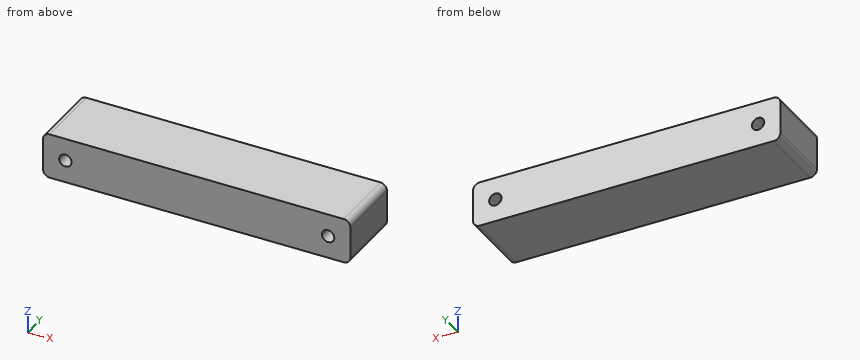
from build123d import *

# Parameters (mm, degrees)
BOSS_EXTRUDE1_DEPTH      = 30.2
M5_CLEARANCE_HOLE1_D     = 5.5
M5_CLEARANCE_HOLE1_DEPTH = 30.2


with BuildPart() as part:
    # Sketch1 → Boss-Extrude1 (new body)
    with BuildSketch(Plane(origin=(0, 0, 0), x_dir=(1, 0, 0), z_dir=(0, 1, 0))):
        with BuildLine():
            Line((65, -10), (-65, -10))
            ThreePointArc((-65, -10), (-67.121320344, -9.121320344), (-68, -7))
            Line((-68, -7), (-68, 7))
            ThreePointArc((-68, 7), (-67.121320344, 9.121320344), (-65, 10))
            Line((-65, 10), (65, 10))
            ThreePointArc((65, 10), (67.121320344, 9.121320344), (68, 7))
            Line((68, 7), (68, -7))
            ThreePointArc((68, -7), (67.121320344, -9.121320344), (65, -10))
        make_face()
    extrude(amount=BOSS_EXTRUDE1_DEPTH)

    # M5 Clearance Hole1
    with Locations(Plane(origin=(0, 30.2, 0), x_dir=(1, 0, 0), z_dir=(0, 1, 0))):
        with Locations((-58.1, 0), (58.1, 0)):
            Hole(M5_CLEARANCE_HOLE1_D / 2, depth=M5_CLEARANCE_HOLE1_DEPTH)


solid = part.part
Check sheet for the modelled part. Datum: model origin and axes. Units: mm. Give positions to 0.01 mm unless a question says otherwise; leave off trailing zeros. Write each loop counter-clockwise with the first axis right and the second up, starting at its lowest first coordinate (ties: lowest second). Pieces come first, ordered by that corner, then holes. Notation, with made-up numbers: (47.5, -24) -> (51.5, -24) arc R34 ccw to (51.5, 13) -> close; hole circle Ø6 at (36, 78.5). An arc over 180 degrees is marked (long way). Write item = value, one per line.
Item 1: Sectioned sample at B-B on x = -58.1. Record the boundary of the cut face in (y, z), and give its area (3 significant figures).
Output:
outline = (0, -10) -> (30.2, -10) -> (30.2, -2.75) -> (0, -2.75) -> close; (0, 2.75) -> (30.2, 2.75) -> (30.2, 10) -> (0, 10) -> close
area = 438 mm^2
Item 2: Scan lines: probe 1 along Z at (x, y) = (58, 20); probe 2 along X at (y, z) = (23, -2.25); probe 3 along X at (y, z) = (27.5, 7.25). Record each from-to range of solid material in increasing order. Write a range as from..to.
Output:
probe_1 = -10..-2.75, 2.75..10
probe_2 = -68..-59.68, -56.52..56.52, 59.68..68
probe_3 = -67.99..67.99
Item 3: Sectioned sample at C-C on y = 18.5. Record the boundary of the cut face in (x, z).
Output:
outline = (-68, -7) arc R3 ccw to (-65, -10) -> (65, -10) arc R3 ccw to (68, -7) -> (68, 7) arc R3 ccw to (65, 10) -> (-65, 10) arc R3 ccw to (-68, 7) -> close; hole circle Ø5.5 at (-58.1, 0); hole circle Ø5.5 at (58.1, 0)
Item 4: Gauge pin test, flat end, axial feed: pin 1 (6.5 mm diameter, centred on x = -58.1, z = 0, fed in from +Y). Record the tip position at first contact, or that the pin passes through.
Output:
pin_1 = 30.2
Item 5: Sectioned sample at A-A on z = 0. Record the boundary of the cut face in (x, y).
Output:
outline = (-68, 0) -> (-60.85, 0) -> (-60.85, 30.2) -> (-68, 30.2) -> close; (-55.35, 0) -> (55.35, 0) -> (55.35, 30.2) -> (-55.35, 30.2) -> close; (60.85, 0) -> (68, 0) -> (68, 30.2) -> (60.85, 30.2) -> close
